from build123d import *

# Parameters (mm, degrees)
CROQUIS1_W              = 30
CROQUIS1_H              = 20
CROQUIS1_R              = 3.25
SALIENTE_EXTRUIR1_DEPTH = 3
CROQUIS3_W              = 1.712937005
CROQUIS3_H              = 20
SALIENTE_EXTRUIR2_DEPTH = 5
REDONDEO1_R             = 4
REDONDEO2_R             = 4


with BuildPart() as part:
    # Croquis1 → Saliente-Extruir1 (new body)
    with BuildSketch(Plane.XY):
        Rectangle(CROQUIS1_W, CROQUIS1_H)
        Circle(CROQUIS1_R, mode=Mode.SUBTRACT)
    extrude(amount=SALIENTE_EXTRUIR1_DEPTH)

    # Croquis3 → Saliente-Extruir2 (add)
    with BuildSketch(Plane.XY.offset(3)):
        with Locations((-14.143531498, 0)):
            Rectangle(CROQUIS3_W, CROQUIS3_H)
        with Locations((14.143531498, 0)):
            Rectangle(CROQUIS3_W, CROQUIS3_H)
    extrude(amount=SALIENTE_EXTRUIR2_DEPTH)

    # Redondeo1
    # the kernel refuses this fillet: 4 mm, written as the material it takes off along each edge
    with BuildSketch(Plane(origin=(13.287062995, 10, 3), x_dir=(0, 0, -1), z_dir=(-1, 0, 0))) as redondeo1_piece_1:
        with BuildLine():
            CenterArc((REDONDEO1_R, REDONDEO1_R), REDONDEO1_R, 180, 90)
            Line((0, REDONDEO1_R), (0, 0))
            Line((0, 0), (REDONDEO1_R, 0))
        make_face()
    extrude(amount=26.574125991, mode=Mode.SUBTRACT)

    # Redondeo2
    # the kernel refuses this fillet: 4 mm, written as the material it takes off along each edge
    with BuildSketch(Plane(origin=(-13.287062995, -10, 3), x_dir=(0, 0, -1), z_dir=(1, 0, 0))) as redondeo2_piece_1:
        with BuildLine():
            CenterArc((REDONDEO2_R, REDONDEO2_R), REDONDEO2_R, 180, 90)
            Line((0, REDONDEO2_R), (0, 0))
            Line((0, 0), (REDONDEO2_R, 0))
        make_face()
    extrude(amount=26.574125991, mode=Mode.SUBTRACT)


solid = part.part
Source: CAD feature listing. Evaluate the final solid. Frame: model axes, mm. A direction names the side the tool comes from. Round coordinates to 2 decimals unless told otherwise and drop trailing zeros. Loops run counter-clockwise (first coordinate to the right, second up) from the corner with the lowest first, then second, coordinate; pieces in that order, holes last. Notation, with made-up numbers: M -21,46 L 36,46 A21 cw 36,72 Z; hole C 0.25,59.25 d7. An arc over 180 degrees is marked long. Answer as CSV lines item,"result".
Q1. Cut plane B-B (x = 0). Return the cut outline in (y, z), plus the area to 3 significant figures.
Verdict:
outline,"M -9.87,0 L -3.25,0 L -3.25,3 L -6,3 A4 ccw Z; M 3.25,0 L 9.87,0 A4 ccw 6,3 L 3.25,3 Z"
area,"33.7 mm^2"
Q2. Cut plane D-D (z = 0.75). Return the cut outline in (x, y), plus the area to 3 significant figures.
Verdict:
outline,"M -15,-10 L -13.29,-10 L -13.29,-9.6 L 13.29,-9.6 L 13.29,-10 L 15,-10 L 15,10 L 13.29,10 L 13.29,9.6 L -13.29,9.6 L -13.29,10 L -15,10 Z; hole C 0,0 d6.5"
area,"545 mm^2"
Q3. Contact query for flat-ended pins moving along their axis: pin 1 (4 mm diameter, centred on x = -1, y = -1, fed in from -Z); pin 2 (9.5 mm diameter, centred on x = 1, y = -2, fed in from +Z). Output: stop coordinate, or through.
Verdict:
pin 1,"stops at z = 0"
pin 2,"stops at z = 3"
Q4. Pull-direction query (X, two-part tool) for faces 4 (the face through (15, 0, 4)), 5 (the face through (-0.2, -8.4, 2.2)), 6 (the face through (14, 10, 4)); classes: +X half, -X half, draft (parallel to the pull), parting line (faces both ways), or undercut.
Verdict:
face 4,"+X half"
face 5,"undercut"
face 6,"draft"
Q5. Cut plane C-C (y = 0). Return the cut outline in (x, z).
Verdict:
outline,"M -15,0 L -3.25,0 L -3.25,3 L -13.29,3 L -13.29,8 L -15,8 Z; M 3.25,0 L 15,0 L 15,8 L 13.29,8 L 13.29,3 L 3.25,3 Z"
Q6. Cut plane A-A (z = 4.25). Return the cut outline in (x, y), plus the area to 3 significant figures.
Verdict:
outline,"M -15,-10 L -13.29,-10 L -13.29,10 L -15,10 Z; M 13.29,-10 L 15,-10 L 15,10 L 13.29,10 Z"
area,"68.5 mm^2"
Q7. Reachability of faces 1 (the face through (-3.1, 1.4, 3)), 2 (the face through (-14, 0, 8)), 3 (the face through (0.2, 8.4, 2.2)) from +Z, -Z, +X, -X, +Y, -Y: full face, straight path, thin tool, end or side. Return the list, or none.
Verdict:
face 1,"+Z, +Y, -Y"
face 2,"+Z, +X, -X, +Y, -Y"
face 3,"+Z, +Y"
Q8. Line query: line 1 along X through (y, z) = (-3.75, 5); line 2 along Z through (x, y) = (-7, 2); line 3 along Y through (x, z) = (0, 2.35). Output: solid intervals per line, ascending.
Verdict:
line 1,"x = -15 to -13.29, 13.29 to 15"
line 2,"z = 0 to 3"
line 3,"y = -8.19 to -3.25, 3.25 to 8.19"
